from build123d import *

# Parameters (mm, degrees)
SKETCH_1_R           = 26
EXTRUDE_1_DEPTH      = 4
SKETCH_2_OUTSIDE_W   = 68.73
SKETCH_2_OUTSIDE_H   = 68.73
SKETCH_2_OUTSIDE_W_2 = 65.720202688
SKETCH_2_OUTSIDE_H_2 = 40
CUT_EXTRUDE_1_DEPTH  = 4
SKETCH_3_R           = 12.5
EXTRUDE_2_DEPTH      = 10
FILLET_1_R           = 1
CUT_EXTRUDE_2_REACH  = 37.665
SKETCH_4_R           = 3
CUT_EXTRUDE_3_REACH  = 36.293
SKETCH_5_R           = 2.5
CHAMFER_1_SIZE       = 1.5


with BuildPart() as part:
    # Эскиз1 → Бобышка-Вытянуть1 (new body)
    with BuildSketch(Plane(origin=(0, 0, 0), x_dir=(1, 0, 0), z_dir=(0, 1, 0))):
        with Locations(Location((0, 0, 0), (0, 0, 270))):
            Circle(SKETCH_1_R)
    extrude(amount=EXTRUDE_1_DEPTH)

    # Эскиз2 outside → Вырез-Вытянуть1 (cut)
    with BuildSketch(Plane(origin=(0, 4, 0), x_dir=(1, 0, 0), z_dir=(0, 1, 0))):
        Rectangle(SKETCH_2_OUTSIDE_W, SKETCH_2_OUTSIDE_H)
        Rectangle(SKETCH_2_OUTSIDE_W_2, SKETCH_2_OUTSIDE_H_2, mode=Mode.SUBTRACT)
    extrude(amount=-CUT_EXTRUDE_1_DEPTH, mode=Mode.SUBTRACT)

    # Эскиз3 → Бобышка-Вытянуть2 (add)
    with BuildSketch(Plane(origin=(0, 4, 0), x_dir=(1, 0, 0), z_dir=(0, 1, 0))):
        with Locations(Location((0, 0, 0), (0, 0, 270))):
            Circle(SKETCH_3_R)
    extrude(amount=EXTRUDE_2_DEPTH)

    # Скругление1
    fillet_1_edges = [part.edges().sort_by_distance(p)[0] for p in [
        (0, 14, -12.5),
    ]]
    fillet(fillet_1_edges, radius=FILLET_1_R)

    # Эскиз4 → Вырез-Вытянуть2 (cut, up to next)
    with BuildSketch(Plane(origin=(0, 14, 0), x_dir=(1, 0, 0), z_dir=(0, 1, 0)), mode=Mode.PRIVATE) as cut_extrude_2_sk1:
        with Locations(Location((0, 0, 0), (0, 0, 270))):
            Circle(SKETCH_4_R)
    cut_extrude_2_tool1 = extrude(cut_extrude_2_sk1.sketch, amount=-CUT_EXTRUDE_2_REACH, mode=Mode.PRIVATE) & part.part
    add(cut_extrude_2_tool1.solids().sort_by_distance((0, 14, 0))[0], mode=Mode.SUBTRACT)

    # Эскиз5 → Вырез-Вытянуть3 (cut, up to next)
    with BuildSketch(Plane(origin=(0, 4, 0), x_dir=(1, 0, 0), z_dir=(0, 1, 0)), mode=Mode.PRIVATE) as cut_extrude_3_sk1:
        with Locations(Location((-15, 15, 0), (0, 0, 270))):
            Circle(SKETCH_5_R)
    cut_extrude_3_tool1 = extrude(cut_extrude_3_sk1.sketch, amount=-CUT_EXTRUDE_3_REACH, mode=Mode.PRIVATE) & part.part
    # Эскиз5 → Вырез-Вытянуть3 (cut, up to next)
    with BuildSketch(Plane(origin=(0, 4, 0), x_dir=(1, 0, 0), z_dir=(0, 1, 0)), mode=Mode.PRIVATE) as cut_extrude_3_sk2:
        with Locations(Location((15, 15, 0), (0, 0, 270))):
            Circle(SKETCH_5_R)
    cut_extrude_3_tool2 = extrude(cut_extrude_3_sk2.sketch, amount=-CUT_EXTRUDE_3_REACH, mode=Mode.PRIVATE) & part.part
    # Эскиз5 → Вырез-Вытянуть3 (cut, up to next)
    with BuildSketch(Plane(origin=(0, 4, 0), x_dir=(1, 0, 0), z_dir=(0, 1, 0)), mode=Mode.PRIVATE) as cut_extrude_3_sk3:
        with Locations(Location((15, -15, 0), (0, 0, 270))):
            Circle(SKETCH_5_R)
    cut_extrude_3_tool3 = extrude(cut_extrude_3_sk3.sketch, amount=-CUT_EXTRUDE_3_REACH, mode=Mode.PRIVATE) & part.part
    # Эскиз5 → Вырез-Вытянуть3 (cut, up to next)
    with BuildSketch(Plane(origin=(0, 4, 0), x_dir=(1, 0, 0), z_dir=(0, 1, 0)), mode=Mode.PRIVATE) as cut_extrude_3_sk4:
        with Locations(Location((-15, -15, 0), (0, 0, 270))):
            Circle(SKETCH_5_R)
    cut_extrude_3_tool4 = extrude(cut_extrude_3_sk4.sketch, amount=-CUT_EXTRUDE_3_REACH, mode=Mode.PRIVATE) & part.part
    add(cut_extrude_3_tool1.solids().sort_by_distance((-15, 4, -15))[0], mode=Mode.SUBTRACT)
    add(cut_extrude_3_tool2.solids().sort_by_distance((15, 4, -15))[0], mode=Mode.SUBTRACT)
    add(cut_extrude_3_tool3.solids().sort_by_distance((15, 4, 15))[0], mode=Mode.SUBTRACT)
    add(cut_extrude_3_tool4.solids().sort_by_distance((-15, 4, 15))[0], mode=Mode.SUBTRACT)

    # Фаска1
    chamfer_1_edges = [part.edges().sort_by_distance(p)[0] for p in [
        (-15, 4, 12.5),
        (15, 4, 12.5),
        (15, 4, -17.5),
        (-15, 4, -17.5),
    ]]
    chamfer(chamfer_1_edges, length=CHAMFER_1_SIZE)


solid = part.part
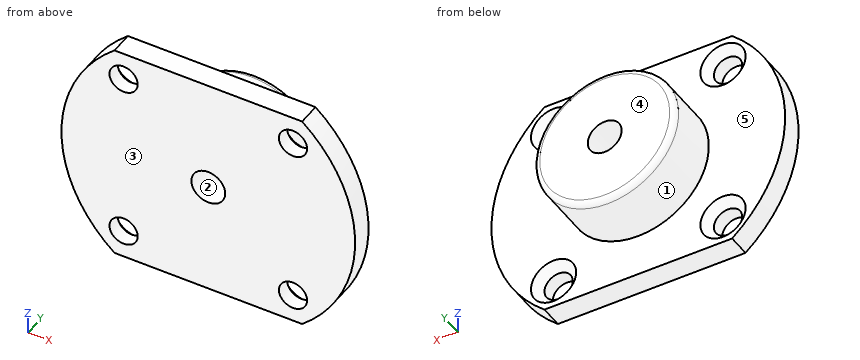
Work out the finished part from the listing and answer in its coordinate system (mm). Face numbers are marked on the shaded views. A direction names the side the tool comes from. Coordinates: 2 decimals unless noted, no trailing zeros. Order: outer loops, then holes, each group sorted by start corner. A loop starts at its lowest first (then second) coordinate and runs counter-clockwise, first axis right, second up. Notation, with made-up numbers: (73, 15.5) - (90, 15.5) arc R8 cw to (90, 28.5) - close; hole circle Ø11 at (-7.75, 66.25). An arc over 180 degrees is marked (long way). Put each result on its own line as item: value. Start each with the question number.
1) Find the intervals of material crossed by line 1 (X direction, y = 1.5, z = -15); line 2 (X direction, y = 0.5, z = 14); line 3 (Z direction, x = -12, y = 3.5), in increasing order. Write a range as from..to.
2) Find section B-B (y = 1.5). Give the vertices of the cut face in (x, z).
3) Flat-ended cylindrical pins translate along their axes: pin 1 (1.5 mm diameter, centred on x = -17, z = -4, fed in from +Y); pin 2 (4 mm diameter, centred on x = -1.5, y = 12.5, fed in from +Z); pin 3 (5 mm diameter, centred on y = 5.5, z = -2, fed in from -X). Find the tip coordinate at first contact, or state that the pin passes through.
4) For the marked faces 4 and 5, determine the directions among +Z, -Z, +X, -X, +Y, -Y from which every point of the face is accessible in a straight line to the end or side of a thin tool.
5) For a pull along X with two mould halves and no side action, classify the marked faces 1, 2 and 3 as released by +X, released by -X, zero draft, split by the parting line, or undercut.
6) Find section D-D (z = 15). Give the vertices of the cut face in (x, y), plus the area to 3 significant figures.
7) Find section C-C (x = 0). Give the vertices of the cut face in (y, z), plus the area to 3 significant figures.
8) Find section A-A (x = -15). Give the vertices of the cut face in (y, z).
Results list:
1. line 1: x = -21.24..-17.5, -12.5..12.5, 17.5..21.24
1. line 2: x = -21.91..-17.29, -12.71..12.71, 17.29..21.91
1. line 3: z = -20..-16.8, -13.2..13.2, 16.8..20
2. outline: (-16.61, -20) - (16.61, -20) arc R26 ccw to (16.61, 20) - (-16.61, 20) arc R26 ccw to start; hole circle Ø5 at (-15, -15); hole circle Ø5 at (-15, 15); hole circle Ø6 at (0, 0); hole circle Ø5 at (15, -15); hole circle Ø5 at (15, 15)
3. pin 1: stops at y = 4
3. pin 2: stops at z = 12.5
3. pin 3: stops at x = -26
4. face 4: +Z, -Z, +X, -X, +Y
4. face 5: +Y
5. face 1: split by the parting line
5. face 2: undercut
5. face 3: zero draft
6. outline: (-21.24, 0) - (-17.5, 0) - (-17.5, 2.5) - (-19, 4) - (-21.24, 4) - close; (-12.5, 0) - (12.5, 0) - (12.5, 2.5) - (11, 4) - (-11, 4) - (-12.5, 2.5) - close; (17.5, 0) - (21.24, 0) - (21.24, 4) - (19, 4) - (17.5, 2.5) - close
6. area: 125 mm^2
7. outline: (0, -20) - (4, -20) - (4, -12.5) - (13, -12.5) arc R1 ccw to (14, -11.5) - (14, -3) - (0, -3) - close; (0, 3) - (14, 3) - (14, 11.5) arc R1 ccw to (13, 12.5) - (4, 12.5) - (4, 20) - (0, 20) - close
7. area: 326 mm^2
8. outline: (0, -20) - (4, -20) - (4, -19) - (2.5, -17.5) - (0, -17.5) - close; (0, -12.5) - (2.5, -12.5) - (4, -11) - (4, 11) - (2.5, 12.5) - (0, 12.5) - close; (0, 17.5) - (2.5, 17.5) - (4, 19) - (4, 20) - (0, 20) - close
